Check sheet for the drawn part. Datum: minimum x, y, z corner. Units: mm. A direction names the side the tool comes from. Round coordinates to 2 decimals unless told otherwise and drop trailing zeros. Order: outer loops, then holes, each group sorted by start corner. A loop starts at its lowest first (then second) coordinate and runs counter-clockwise, first axis right, second up. Notation, with made-up numbers: (24.25, 17.25) -> (73.25, 17.25) arc R21 ccw to (73.25, 28.25) -> close; hole circle Ø2 at (86, 69). An arc over 180 degrees is marked (long way). Answer in a Markdown table with one row per item.
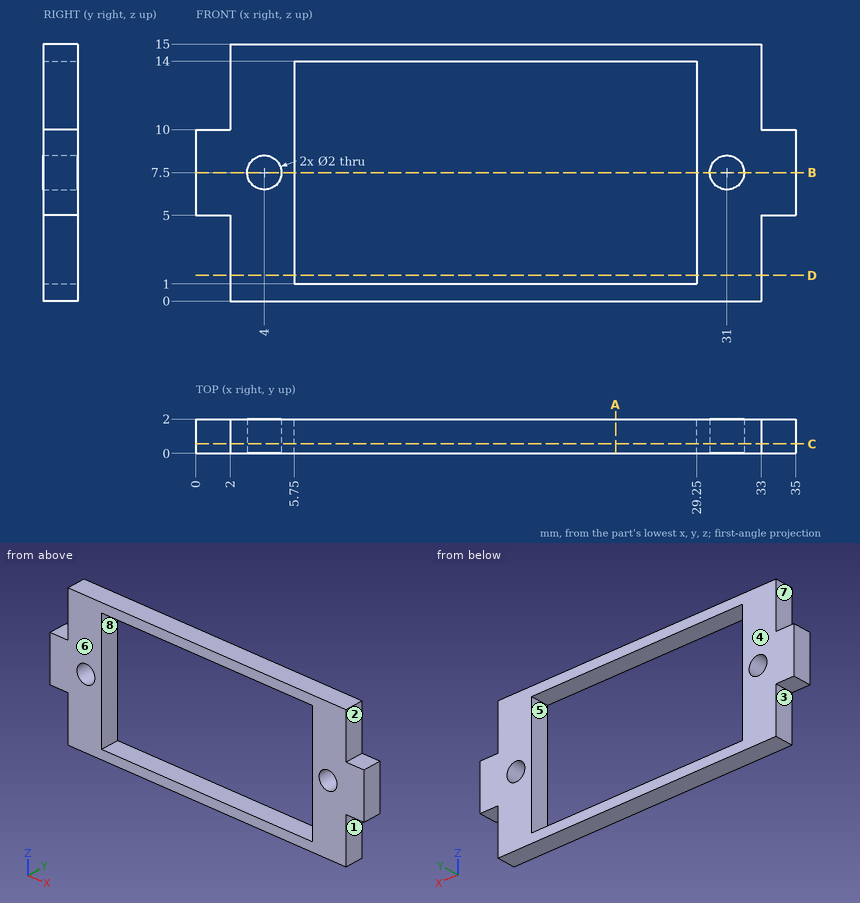
(1) Scan lines: probe 1 along X at (y, z) = (0.7, 7.5); probe 2 along X at (y, z) = (1.95, 5.25); probe 3 along X at (y, z) = (0.6, 3.75). Record each from-to range of solid material in increasing order. Write a range as from..to.
Solutions:
| item | result |
|---|---|
| probe 1 | 0..3, 5..5.75, 29.25..30, 32..35 |
| probe 2 | 0..5.75, 29.25..35 |
| probe 3 | 2..5.75, 29.25..33 |
(2) Section check A-A on x = 24.5. Record the boundary of the cut face in (y, z).
Solutions:
| item | result |
|---|---|
| outline | (0, 0) -> (2, 0) -> (2, 1) -> (0, 1) -> close; (0, 14) -> (2, 14) -> (2, 15) -> (0, 15) -> close |
(3) Draft check along X on the marked faces 6, 7 and 8. Enter one of: pulls with the +X half, pulls with the -X half, needs draft (parallel to the pull), parting line crosses it, or undercut.
Solutions:
| item | result |
|---|---|
| face 6 | needs draft |
| face 7 | pulls with the -X half |
| face 8 | undercut |
(4) Section check C-C on y = 0.55. Record the boundary of the cut face in (x, z).
Solutions:
| item | result |
|---|---|
| outline | (0, 5) -> (2, 5) -> (2, 0) -> (33, 0) -> (33, 5) -> (35, 5) -> (35, 10) -> (33, 10) -> (33, 15) -> (2, 15) -> (2, 10) -> (0, 10) -> close; hole circle Ø2 at (4, 7.5); hole (5.75, 1) -> (29.25, 1) -> (29.25, 14) -> (5.75, 14) -> close; hole circle Ø2 at (31, 7.5) |
(5) Depth check by flat-ended pin: pin 1 Ø1 at (x, y) = (34, 1) entering from -Z; pin 2 Ø1 at (y, z) = (1, 2) entering from +X. Enter the tip coordinate at first touch or a pass-through.
Solutions:
| item | result |
|---|---|
| pin 1 | z = 5 |
| pin 2 | x = 33 |
(6) Section check D-D on z = 1.5. Record the boundary of the cut face in (x, y), plus the area to 3 significant figures.
Solutions:
| item | result |
|---|---|
| outline | (2, 0) -> (5.75, 0) -> (5.75, 2) -> (2, 2) -> close; (29.25, 0) -> (33, 0) -> (33, 2) -> (29.25, 2) -> close |
| area | 15.0 mm^2 |
(7) Tool access check on the marked faces 1, 2, 3, 4 and 5. Record the directions out of +Z, -Z, +X, -X, +Y, -Y that give a thin tool (end or side, any length) a straight path to the whole face; none if there is none.
Solutions:
| item | result |
|---|---|
| face 1 | -Z, +X, +Y, -Y |
| face 2 | +Z, +X, +Y, -Y |
| face 3 | -Z, -X, +Y, -Y |
| face 4 | +Z, -Z, +X, -X, +Y |
| face 5 | +Y, -Y |
(8) Section check B-B on z = 7.5. Record the boundary of the cut face in (x, y), plus the area to 3 significant figures.
Solutions:
| item | result |
|---|---|
| outline | (0, 0) -> (3, 0) -> (3, 2) -> (0, 2) -> close; (5, 0) -> (5.75, 0) -> (5.75, 2) -> (5, 2) -> close; (29.25, 0) -> (30, 0) -> (30, 2) -> (29.25, 2) -> close; (32, 0) -> (35, 0) -> (35, 2) -> (32, 2) -> close |
| area | 15.0 mm^2 |
